Work out the finished part from the listing and answer in its coordinate system (mm). Coordinates: 2 decimals unless noted, no trailing zeros. Loops run counter-clockwise (first coordinate to the right, second up) from the corner with the lowest first, then second, coordinate; pieces in that order, holes last. Notation, with made-up numbers: (59.25, 34) -> (67.25, 34) arc R25 ccw to (67.25, 72) -> close; hole circle Ø1 at (13.25, 83.5). An arc over 180 degrees is marked (long way). Use a Markdown table: item, result. Add a question column.
Autodesk Inventor part; units mm, degrees
ref_plane "Work Plane1" through (0, 86, 164.5) normal (0, 1, 0) x (1, 0, 0)
ref_plane "YZ Plane" through (0, 0, 0) normal (1, 0, 0) x (0, 1, 0)
ref_plane "XZ Plane" through (0, 0, 0) normal (0, 1, 0) x (-1, 0, 0)
ref_plane "Work Plane1" through (0, 86, 164.5) normal (0, 1, 0) x (1, 0, 0)
sketch "Sketch7" plane through (0, 86, 164.5) normal (0, 1, 0) x (1, 0, 0)
  line L0 (-3, 170.5) -> (5, 170.5) construction
  line L1 (-3, 170.5) -> (-3, -3) construction
  line L2 (173.5, -3) -> (-3, -3) construction
  line L3 (173.5, 170.5) -> (173.5, -3) construction
  line L4 (165.5, 170.5) -> (173.5, 170.5) construction
  line L5 (165.5, 170.5) -> (165.5, 167.3) construction
  line L6 (170.5, 167.3) -> (165.5, 167.3) construction
  line L7 (170.5, 167.3) -> (170.5, 164.5) construction
  line L8 (170.5, 164.5) -> (165.5, 164.5) construction
  line L9 (165.5, 164.5) -> (165.5, 160.5) construction
  line L10 (170.5, 160.5) -> (165.5, 160.5) construction
  line L11 (170.5, 160.5) -> (170.5, 0) construction
  line L12 (170.5, 0) -> (0, 0) construction
  line L13 (0, 0) -> (0, 160.5) construction
  line L14 (5, 160.5) -> (0, 160.5) construction
  line L15 (5, 164.5) -> (5, 160.5) construction
  line L16 (5, 164.5) -> (0, 164.5) construction
  line L17 (0, 164.5) -> (0, 167.3) construction
  line L18 (5, 167.3) -> (0, 167.3) construction
  line L19 (5, 170.5) -> (5, 167.3) construction
  line L20 (165.3, 160.3) -> (165.3, 164.7) construction
  line L21 (165.3, 164.7) -> (170.3, 164.7) construction
  line L22 (170.3, 164.7) -> (170.3, 167.1) construction
  line L23 (170.3, 167.1) -> (165.3, 167.1) construction
  line L24 (165.3, 167.1) -> (165.3, 170.7) construction
  line L25 (165.3, 170.7) -> (173.7, 170.7) construction
  line L26 (173.7, 170.7) -> (173.7, -3.2) construction
  line L27 (173.7, -3.2) -> (-3.2, -3.2) construction
  line L28 (-3.2, -3.2) -> (-3.2, 170.7) construction
  line L29 (-3.2, 170.7) -> (5.2, 170.7) construction
  line L30 (5.2, 170.7) -> (5.2, 167.1) construction
  line L31 (5.2, 167.1) -> (0.2, 167.1) construction
  line L32 (0.2, 167.1) -> (0.2, 164.7) construction
  line L33 (0.2, 164.7) -> (5.2, 164.7) construction
  line L34 (5.2, 164.7) -> (5.2, 160.3) construction
  line L35 (5.2, 160.3) -> (0.2, 160.3) construction
  line L36 (0.2, 160.3) -> (0.2, 0.2) construction
  line L37 (0.2, 0.2) -> (170.3, 0.2) construction
  line L38 (170.3, 0.2) -> (170.3, 160.3) construction
  line L39 (170.3, 160.3) -> (165.3, 160.3) construction
  line L40 (170.3, 160.3) -> (0.2, 160.3)
  line L41 (0.2, 160.3) -> (0.2, 0.2)
  line L42 (0.2, 0.2) -> (170.3, 0.2)
  line L43 (170.3, 0.2) -> (170.3, 160.3)
  point P0 (0, 164.5)
  dimension "d18" = 0.2
extrude "Extrusion7" add sketch "Sketch7" along normal blind 3
sketch "Sketch8" plane through (0, 89, 164.5) normal (0, 1, 0) x (1, 0, 0)
  line L0 (-3, 170.5) -> (5, 170.5) construction
  line L1 (-3, 170.5) -> (-3, -3) construction
  line L2 (173.5, -3) -> (-3, -3) construction
  line L3 (173.5, 170.5) -> (173.5, -3) construction
  line L4 (165.5, 170.5) -> (173.5, 170.5) construction
  line L5 (165.5, 170.5) -> (165.5, 167.3) construction
  line L6 (170.5, 167.3) -> (165.5, 167.3) construction
  line L7 (170.5, 167.3) -> (170.5, 164.5) construction
  line L8 (170.5, 164.5) -> (165.5, 164.5) construction
  line L9 (165.5, 164.5) -> (165.5, 160.5) construction
  line L10 (170.5, 160.5) -> (165.5, 160.5) construction
  line L11 (170.5, 160.5) -> (170.5, 0) construction
  line L12 (170.5, 0) -> (0, 0) construction
  line L13 (0, 0) -> (0, 160.5) construction
  line L14 (5, 160.5) -> (0, 160.5) construction
  line L15 (5, 164.5) -> (5, 160.5) construction
  line L16 (5, 164.5) -> (0, 164.5) construction
  line L17 (0, 164.5) -> (0, 167.3) construction
  line L18 (5, 167.3) -> (0, 167.3) construction
  line L19 (5, 170.5) -> (5, 167.3) construction
  line L20 (173.5, 170.5) -> (-3, 170.5) construction
  line L21 (-3, 170.5) -> (-3, -3) construction
  line L22 (-3, -3) -> (173.5, -3) construction
  line L23 (173.5, -3) -> (173.5, 170.5) construction
  line L24 (173.5, 170.5) -> (-3, 170.5)
  line L25 (-3, 170.5) -> (-3, -3)
  line L26 (-3, -3) -> (173.5, -3)
  line L27 (173.5, -3) -> (173.5, 170.5)
  point P0 (0, 164.5)
extrude "Extrusion8" add sketch "Sketch8" along normal blind 3
sketch "Sketch9" plane through (0, 92, 164.5) normal (0, 1, 0) x (1, 0, 0)
  line L0 (-3, 170.5) -> (-3, -3) construction
  line L1 (-3, -3) -> (173.5, -3) construction
  line L2 (173.5, -3) -> (173.5, 170.5) construction
  line L3 (173.5, 170.5) -> (-3, 170.5) construction
  line L4 (109.75, 30) -> (60.75, 30) construction
  line L5 (52.75, 22) -> (52.75, 22) construction
  line L6 (60.75, 14) -> (109.75, 14) construction
  line L7 (117.75, 22) -> (117.75, 22) construction
  line L8 (117.75, 30) -> (52.75, 14) construction
  line L9 (52.75, 30) -> (117.75, 14) construction
  line L10 (85.25, 22) -> (85.25, -3) construction
  arc A0 (109.75, 14) -> (117.75, 22) centre (109.75, 22) ccw construction
  arc A1 (52.75, 22) -> (60.75, 14) centre (60.75, 22) ccw construction
  arc A2 (60.75, 30) -> (52.75, 22) centre (60.75, 22) ccw construction
  arc A3 (117.75, 22) -> (109.75, 30) centre (109.75, 22) ccw construction
  line L11 (109.75, 30) -> (60.75, 30) construction
  line L12 (60.75, 30) -> (60.75, 14) construction
  line L13 (60.75, 14) -> (109.75, 14) construction
  line L14 (109.75, 14) -> (109.75, 30) construction
  line L15 (109.75, 30) -> (60.75, 30)
  line L16 (60.75, 14) -> (109.75, 14)
  arc A4 (109.75, 14) -> (109.75, 30) centre (109.75, 22) ccw
  arc A5 (60.75, 30) -> (60.75, 14) centre (60.75, 22) ccw
  point P0 (0, 164.5)
  dimension "d23" = 65
  dimension "d24" = 16
  dimension "d25" = 25
  dimension "d26" = 8
extrude "Extrusion9" cut sketch "Sketch9" against normal blind 6
fillet "Fillet1" radius 3 8 edges at (52.75, 92, 142.5) (85.25, 92, 134.5) (117.75, 92, 142.5) (85.25, 92, 150.5) (117.75, 86, 142.5) (85.25, 86, 134.5) (52.75, 86, 142.5) (85.25, 86, 150.5)
properties part number "Lid"
Item 1: Section D-D (y = 87.2) is taken. Determine the outline of the cut face in (x, z).
Item 2: Section C-C (z = 30) is taken. Determine the outline of the cut face in (x, y).
Item 3: Given pin 1 (2.5 mm diameter, centred on x = 90.5, y = 87, fed in from -Z); pin 2 (1.5 mm diameter, centred on x = 60.5, y = 87.5, fed in from +Z); pin 3 (0.9 mm diameter, centred on y = 87.5, z = 113, fed in from +X), each flat-ended and moving along its own axis, determine where each tip first touches the part or whether it passes through.
Item 4: Find the intervals of material crossed by probe 1 along Z at (x, y) = (100, 89.2); probe 2 along X at (y, z) = (87.95, 70.5); probe 3 along Z at (x, y) = (67.5, 86.25), in increasing order.
Output:
| question | item | result |
|---|---|---|
| 1 | outline | (0.2, 4.2) -> (170.3, 4.2) -> (170.3, 164.3) -> (0.2, 164.3) -> close; hole (60.75, 133.9) -> (109.75, 133.9) arc R8.6 ccw to (109.75, 151.1) -> (60.75, 151.1) arc R8.6 ccw to start |
| 2 | outline | (-3, 89) -> (0.2, 89) -> (0.2, 86) -> (170.3, 86) -> (170.3, 89) -> (173.5, 89) -> (173.5, 92) -> (-3, 92) -> close |
| 3 | pin 1 | stops at z = 4.2 |
| 3 | pin 2 | stops at z = 164.3 |
| 3 | pin 3 | stops at x = 170.3 |
| 4 | probe 1 | z = -6 to 134.49, 150.51 to 167.5 |
| 4 | probe 2 | x = 0.2 to 170.3 |
| 4 | probe 3 | z = 4.2 to 132.7, 152.3 to 164.3 |
